Check sheet for the modelled part. Datum: model origin and axes. Units: mm. A direction names the side the tool comes from. Round coordinates to 2 decimals unless told otherwise and drop trailing zeros. Write each loop counter-clockwise with the first axis right and the second up, starting at its lowest first coordinate (ties: lowest second). Pieces come first, ordered by that corner, then holes. Notation, with made-up numbers: M 77.25,41 L 88.25,41 A11 ccw 88.25,58 Z; hole C 72,51.25 d1. An arc over 180 degrees is marked long. Answer in a Markdown table with one row per item.
```python
from build123d import *

# Parameters (mm, degrees)
BOSS_EXTRUDE1_DEPTH     = 146.875
SKETCH2_W               = 273.75
SKETCH2_H               = 213.261995914
CUT_EXTRUDE1_DEPTH      = 708.854574743
FILLET1_R               = 10
FILLET2_R               = 20
SKETCH3_R               = 25
BOSS_EXTRUDE2_DEPTH     = 273.75
BOSS_EXTRUDE3_DEPTH     = 20
SKETCH5_R               = 51.111383935
SKETCH5_R_2             = 17.147302995
CUT_EXTRUDE2_DEPTH      = 20
CUT_EXTRUDE2_TAPER      = 45
CUT_EXTRUDE3_DEPTH      = 495.366464437
CUT_EXTRUDE3_DEPTH_BACK = 495.366464437
CUT_EXTRUDE4_DEPTH      = 417.900952607
CUT_EXTRUDE4_DEPTH_BACK = 10
FILLET3_R               = 20


with BuildPart() as part:
    # Sketch1 → Boss-Extrude1 (new, symmetric)
    with BuildSketch(Plane.XY):
        Polygon((-333.43, 0), (333.43, 0), (333.43, -80.23), (196.11, -186.50354892), (-196.11, -186.50354892), (-333.43, -80.23), align=None)
    extrude(amount=BOSS_EXTRUDE1_DEPTH, both=True)

    # Sketch2 → Cut-Extrude1 (cut, through all)
    with BuildSketch(Plane(origin=(333.43, 0, 0), x_dir=(0, 0, -1), z_dir=(1, 0, 0))):
        with Locations((0, -69.872550963)):
            Rectangle(SKETCH2_W, SKETCH2_H)
    extrude(amount=-CUT_EXTRUDE1_DEPTH, mode=Mode.SUBTRACT)

    # Fillet1
    fillet1_edges = [part.edges().sort_by_distance(p)[0] for p in [
        (0, -176.50354892, -136.875),
        (0, -176.50354892, 136.875),
    ]]
    fillet(fillet1_edges, radius=FILLET1_R)

    # Fillet2
    fillet2_edges = [part.edges().sort_by_distance(p)[0] for p in [
        (0, -186.50354892, -146.875),
        (0, -186.50354892, 146.875),
    ]]
    fillet(fillet2_edges, radius=FILLET2_R)

    # Sketch3 → Boss-Extrude2 (add)
    with BuildSketch(Plane(origin=(0, 0, 136.875), x_dir=(-1, 0, 0), z_dir=(0, 0, -1))):
        with Locations(Location((0, -80.23, 0), (0, 0, 270))):
            Circle(SKETCH3_R)
    extrude(amount=BOSS_EXTRUDE2_DEPTH)

    # Sketch4 → Boss-Extrude3 (add)
    with BuildSketch(Plane.XY.offset(146.875)):
        Polygon((0, -100.03), (17.147302995, -90.13), (17.147302995, -70.33), (0, -60.43), (-17.147302995, -70.33), (-17.147302995, -90.13), align=None)
    boss_extrude3 = extrude(amount=BOSS_EXTRUDE3_DEPTH)

    # Sketch5 → Cut-Extrude2 (cut)
    with BuildSketch(Plane.XY.offset(166.875)):
        with Locations((0, -80.23)):
            Circle(SKETCH5_R)
        with Locations((0, -80.23)):
            Circle(SKETCH5_R_2, mode=Mode.SUBTRACT)
    cut_extrude2 = extrude(amount=-CUT_EXTRUDE2_DEPTH, taper=CUT_EXTRUDE2_TAPER, mode=Mode.SUBTRACT)

    # Mirror1: Boss-Extrude3, Cut-Extrude2 across plane
    add(boss_extrude3.mirror(Plane.XY))
    add(cut_extrude2.mirror(Plane.XY), mode=Mode.SUBTRACT)

    # Sketch6 → Cut-Extrude3 (cut, two sides: drawn at the far end of the back side and taken through both)
    with BuildSketch(Plane.XY.offset(146.875).offset(-CUT_EXTRUDE3_DEPTH_BACK)):
        with BuildLine():
            Line((-303.5, -37.26), (-303.5, -52.66))
            ThreePointArc((-303.5, -52.66), (-302.527520815, -56.961612248), (-299.799226414, -60.426578821))
            Line((-299.799226414, -60.426578821), (-185.419226414, -153.196578821))
            ThreePointArc((-185.419226414, -153.196578821), (-182.461721995, -154.855120376), (-179.12, -155.43))
            Line((-179.12, -155.43), (-67, -155.43))
            ThreePointArc((-67, -155.43), (-59.928932188, -152.501067812), (-57, -145.43))
            Line((-57, -145.43), (-57, -37.26))
            ThreePointArc((-57, -37.26), (-59.928932188, -30.188932188), (-67, -27.26))
            Line((-67, -27.26), (-293.5, -27.26))
            ThreePointArc((-293.5, -27.26), (-300.571067812, -30.188932188), (-303.5, -37.26))
        make_face()
        with BuildLine():
            Line((57, -145.43), (57, -37.26))
            ThreePointArc((57, -37.26), (59.928932188, -30.188932188), (67, -27.26))
            Line((67, -27.26), (293.5, -27.26))
            ThreePointArc((293.5, -27.26), (300.571067812, -30.188932188), (303.5, -37.26))
            Line((303.5, -37.26), (303.5, -52.66))
            ThreePointArc((303.5, -52.66), (302.527520815, -56.961612248), (299.799226414, -60.426578821))
            Line((299.799226414, -60.426578821), (185.419226414, -153.196578821))
            ThreePointArc((185.419226414, -153.196578821), (182.461721995, -154.855120376), (179.12, -155.43))
            Line((179.12, -155.43), (67, -155.43))
            ThreePointArc((67, -155.43), (59.928932188, -152.501067812), (57, -145.43))
        make_face()
    extrude(amount=CUT_EXTRUDE3_DEPTH + CUT_EXTRUDE3_DEPTH_BACK, mode=Mode.SUBTRACT)

    # Sketch7 → Cut-Extrude4 (cut, two sides: drawn at the far end of the back side and taken through both)
    with BuildSketch(Plane.XZ.offset(186.50354892).offset(-CUT_EXTRUDE4_DEPTH_BACK)):
        with BuildLine():
            Line((166.11, 99), (-166.11, 99))
            ThreePointArc((-166.11, 99), (-173.181067812, 96.071067812), (-176.11, 89))
            Line((-176.11, 89), (-176.11, -89))
            ThreePointArc((-176.11, -89), (-173.181067812, -96.071067812), (-166.11, -99))
            Line((-166.11, -99), (166.11, -99))
            ThreePointArc((166.11, -99), (173.181067812, -96.071067812), (176.11, -89))
            Line((176.11, -89), (176.11, 89))
            ThreePointArc((176.11, 89), (173.181067812, 96.071067812), (166.11, 99))
        make_face()
    extrude(amount=CUT_EXTRUDE4_DEPTH + CUT_EXTRUDE4_DEPTH_BACK, mode=Mode.SUBTRACT)

    # Fillet3
    fillet3_edges = [part.edges().sort_by_distance(p)[0] for p in [
        (-333.43, -80.23, 141.875),
        (-333.43, 0, 141.875),
        (333.43, 0, 141.875),
        (333.43, -80.23, 141.875),
        (-333.43, -80.23, -141.875),
        (-333.43, 0, -141.875),
        (333.43, 0, -141.875),
        (333.43, -80.23, -141.875),
    ]]
    fillet(fillet3_edges, radius=FILLET3_R)


solid = part.part
```
1. Go/stop test with flat-tipped pins: pin 1 (3 mm diameter, centred on x = 146.5, z = -141, fed in from -Y); pin 2 (10 mm diameter, centred on y = -78.5, z = -157, fed in from -X); pin 3 (3 mm diameter, centred on x = 48, y = -183, fed in from +Z). Record where each tip stops, or that it passes through.
Found:
| item | result |
|---|---|
| pin 1 | stops at y = -182.02 |
| pin 2 | stops at x = -17.15 |
| pin 3 | stops at z = 140.11 |
2. Section check B-B, the plane x = 117. Record the cut outline in (y, z) (3 decimals).
Found:
| item | result |
|---|---|
| outline | M -186.504,-126.875 A20 ccw -166.504,-146.875 L -155.43,-146.875 L -155.43,-136.875 L -166.504,-136.875 A10 cw -176.504,-126.875 L -176.504,-99 L -186.504,-99 Z; M -186.504,99 L -176.504,99 L -176.504,126.875 A10 cw -166.504,136.875 L -155.43,136.875 L -155.43,146.875 L -166.504,146.875 A20 ccw -186.504,126.875 Z; M -27.26,-146.875 L 0,-146.875 L 0,-136.875 L -27.26,-136.875 Z; M -27.26,136.875 L 0,136.875 L 0,146.875 L -27.26,146.875 Z |
3. Access from +Z, -Z, +X, -X, +Y, -Y to the whole of each face (thin tool, end or side, straight path). Record for faces 1 (the face through (-243.41, -106.16, 141.8)), 2 (the face through (-8.45, -65.31, 156.74)), 3 (the face through (-8.694, -95.011, 156.735)).
Found:
| item | result |
|---|---|
| face 1 | +Z, -Z |
| face 2 | +Z, -X, +Y |
| face 3 | +Z, -X, -Y |
4. Scan lines: L1, parallel to Z at x = 257.5, y = -96 (3 decimals); L2, parallel to X at y = -81, z = -127.5; L3, parallel to Z at x = -19.5, y = -88 (3 decimals). Record each from-to range of solid material in increasing order.
Found:
| item | result |
|---|---|
| L1 | z = -146.875 to -136.875, 136.875 to 146.875 |
| L2 | x = -24.99 to 24.99 |
| L3 | z = -146.875 to 146.875 |
5. Section check A-A, the plane z = -56. Record the cut outline in (x, y), and give its area (3 significant figures).
Found:
| item | result |
|---|---|
| outline | M -209.03,-176.5 L -196.11,-186.5 L -176.11,-186.5 L -176.11,-176.5 Z; C 0,-80.23 d50; M 176.11,-186.5 L 196.11,-186.5 L 209.03,-176.5 L 176.11,-176.5 Z |
| area | 2,490 mm2 |
6. Section check C-C, the plane y = -112. Record the cut outline in (x, z) (3 decimals).
Found:
| item | result |
|---|---|
| outline | M -292.379,-146.875 L -236.212,-146.875 L -236.212,-136.875 L -292.379,-136.875 Z; M -292.379,136.875 L -236.212,136.875 L -236.212,146.875 L -292.379,146.875 Z; M -57,-146.875 L 57,-146.875 L 57,-136.875 L -57,-136.875 Z; M -57,136.875 L 57,136.875 L 57,146.875 L -57,146.875 Z; M 236.212,-146.875 L 292.379,-146.875 L 292.379,-136.875 L 236.212,-136.875 Z; M 236.212,136.875 L 292.379,136.875 L 292.379,146.875 L 236.212,146.875 Z |
7. Draft check along Y on faces 4 (the face through (243.41, -106.16, -141.94)), 5 (the face through (327.727, -6.014, -141.945)), 6 (the face through (208.409, -176.985, 0.685)). Enter one of: +Y half, -Y half, draft (parallel to the pull), parting line (faces both ways), or undercut.
Found:
| item | result |
|---|---|
| face 4 | undercut |
| face 5 | +Y half |
| face 6 | -Y half |
